from build123d import *

# Parameters (mm, degrees)
SKETCH_1_W          = 69
SKETCH_1_H          = 30
EXTRUDE_1_DEPTH     = 43
SKETCH_3_W          = 63
SKETCH_3_H          = 10
CUT_EXTRUDE_2_DEPTH = 41
SKETCH_4_W          = 69
SKETCH_4_H          = 17
CUT_EXTRUDE_3_DEPTH = 41
SKETCH_5_R          = 2.1
CUT_EXTRUDE_4_DEPTH = 56.643957444
SKETCH_9_W          = 55
SKETCH_9_H          = 30
CUT_EXTRUDE_5_DEPTH = 58.690987164
FILLET_1_R          = 3
FILLET_2_R          = 2
FILLET_3_R          = 1
SKETCH_10_W         = 8
SKETCH_10_H         = 30
CUT_EXTRUDE_6_DEPTH = 83.674058809
FILLET_4_R          = 1
FILLET_5_R          = 1


with BuildPart() as part:
    # 草图1 → 凸台-拉伸1 (new body)
    with BuildSketch(Plane(origin=(0, 0, 0), x_dir=(1, 0, 0), z_dir=(0, 1, 0))):
        Rectangle(SKETCH_1_W, SKETCH_1_H)
    extrude(amount=EXTRUDE_1_DEPTH)

    # 草图3 → 切除-拉伸2 (cut)
    with BuildSketch(Plane(origin=(0, 43, 0), x_dir=(1, 0, 0), z_dir=(0, 1, 0))):
        with Locations((-0.5, -10)):
            Rectangle(SKETCH_3_W, SKETCH_3_H)
    extrude(amount=-CUT_EXTRUDE_2_DEPTH, mode=Mode.SUBTRACT)

    # 草图4 → 切除-拉伸3 (cut)
    with BuildSketch(Plane(origin=(0, 0, 0), x_dir=(-1, 0, 0), z_dir=(0, -1, 0))):
        with Locations((0, 6.5)):
            Rectangle(SKETCH_4_W, SKETCH_4_H)
    extrude(amount=-CUT_EXTRUDE_3_DEPTH, mode=Mode.SUBTRACT)

    # 草图5 → 切除-拉伸4 (cut, through all)
    with BuildSketch(Plane(origin=(0, 41, 0), x_dir=(-1, 0, 0), z_dir=(0, -1, 0))):
        with Locations(Location((26.5, 7, 0), (0, 0, 90))):
            Circle(SKETCH_5_R)
    cut_extrude_4 = extrude(amount=-CUT_EXTRUDE_4_DEPTH, mode=Mode.SUBTRACT)

    # 镜向1: 切除-拉伸4 across plane
    add(cut_extrude_4.mirror(Plane.ZY), mode=Mode.SUBTRACT)

    # 草图9 → 切除-拉伸5 (cut, through all)
    with BuildSketch(Plane(origin=(0, 0, 2), x_dir=(-1, 0, 0), z_dir=(0, 0, -1))):
        with Locations((0, 20)):
            Rectangle(SKETCH_9_W, SKETCH_9_H)
    extrude(amount=-CUT_EXTRUDE_5_DEPTH, mode=Mode.SUBTRACT)

    # 圆角1
    fillet_1_edges = [part.edges().sort_by_distance(p)[0] for p in [
        (-27.5, 35, 3.5),
        (-27.5, 5, 3.5),
        (27.5, 5, 3.5),
        (27.5, 35, 3.5),
    ]]
    fillet(fillet_1_edges, radius=FILLET_1_R)

    # 圆角2
    fillet_2_edges = [part.edges().sort_by_distance(p)[0] for p in [
        (-34.5, 0, 8.5),
        (34.5, 0, 8.5),
        (-34.5, 42, -15),
        (34.5, 42, -15),
    ]]
    fillet(fillet_2_edges, radius=FILLET_2_R)

    # 圆角3
    fillet_3_edges = [part.edges().sort_by_distance(p)[0] for p in [
        (-32, 2, 10),
        (31, 2, 10),
    ]]
    fillet(fillet_3_edges, radius=FILLET_3_R)

    # 草图10 → 切除-拉伸6 (cut, through all)
    with BuildSketch(Plane.ZY.offset(34.5)):
        with Locations((6, 20.5)):
            Rectangle(SKETCH_10_W, SKETCH_10_H)
    extrude(amount=-CUT_EXTRUDE_6_DEPTH, mode=Mode.SUBTRACT)

    # 圆角4
    fillet_4_edges = [part.edges().sort_by_distance(p)[0] for p in [
        (31, 39.25, 5),
        (-32, 39.25, 5),
        (-33.25, 35.5, 10),
        (32.75, 35.5, 10),
        (32.75, 5.5, 10),
        (-33.25, 5.5, 10),
    ]]
    fillet(fillet_4_edges, radius=FILLET_4_R)

    # 圆角5
    fillet_5_edges = [part.edges().sort_by_distance(p)[0] for p in [
        (0, 0, 2),
        (33.914213562, 0.585786438, 2),
        (-33.914213562, 0.585786438, 2),
        (-34.5, 3.75, 2),
        (34.5, 3.75, 2),
        (-34.5, 38.25, 2),
        (34.5, 38.25, 2),
    ]]
    fillet(fillet_5_edges, radius=FILLET_5_R)


solid = part.part
Geometry: final body of the model. Coordinates: model frame, mm. A direction names the side the tool comes from. Round coordinates to 2 decimals unless told otherwise and drop trailing zeros. Loops run counter-clockwise (first coordinate to the right, second up) from the corner with the lowest first, then second, coordinate; pieces in that order, holes last.
Q1. Pin query (flat end, axial travel): P1, Ø14.5, axis at x = -11, z = -7.5, coming from the -Y side; P2, Ø5, axis at x = 12, y = 4, coming from the -Z side; P3, Ø1, axis at x = 33, y = 26, coming from the -Z side. Return the tip coordinate at first contact, or that it passes through.
Q2. Pull-direction query (X, two-part tool) for faces 4 (the cylindrical face through (33.93, 42.01, -14.4)), 5 (the flat face through (0, 43, -4)), 6 (the flat face through (31, 23, 12)); classes: released by +X, released by -X, zero draft, split by the parting line, or undercut.
Q3. Section A-A on x = -22. Return loops of the section in (y, z).
Q4. Material intervals for L1, parallel to X at y = 42, z = -7; L2, parallel to Z at x = 26.5, y = 42.35; L3, parallel to Y at x = -13, z = 0.5, sorted ascending.
Q5. Section B-B on z = -7. Return loops of the section in (x, y).
Q6. Section D-D on z = -1.5. Return loops of the section in (x, y).
Q7. Section C-C on y = 31.5. Return loops of the section in (x, z), plus the area to 3 significant figures.
Q8. Access query for faces 1 (the flat face through (0, 41, -6)), 2 (the flat face through (0, 5, 3)), 3 (the flat face through (-1, 2, 10)). Directions: +Z, -Z, +X, -X, +Y, -Y. A direction counts if a zero-diameter tool reaches every point of the face in a straight line with its end or side. Return the directions, or none.
Evaluation:
1. P1: stops at y = 41
1. P2: stops at z = 2
1. P3: stops at z = 10
2. face 4: released by +X
2. face 5: zero draft
2. face 6: undercut
3. outline: (0, 3) arc R1 ccw to (1, 2) - (5, 2) - (5, 5) - (2, 5) - (2, 15) - (0, 15) - close; (35.5, 2) - (41, 2) - (41, -15) - (43, -15) - (43, 5) - (35.5, 5) - close
4. L1: x = -34.5 to -28.6, -24.4 to 24.4, 28.6 to 34.5
4. L2: z = -15 to -9.1, -4.9 to 5
4. L3: y = 41 to 43
5. outline: (-34.5, 41) - (-28.6, 41) - (-28.6, 43) - (-34.5, 43) - close; (-24.4, 41) - (24.4, 41) - (24.4, 43) - (-24.4, 43) - close; (28.6, 41) - (34.5, 41) - (34.5, 43) - (28.6, 43) - close
6. outline: (-34.5, 41) - (34.5, 41) - (34.5, 43) - (-34.5, 43) - close
7. outline: (-34.5, 10) - (-32, 10) - (-32, 15) - (-34.5, 15) - close; (31, 10) - (34.5, 10) - (34.5, 15) - (31, 15) - close
7. area: 30.0 mm2
8. face 1: -Z, +X, -X, -Y
8. face 2: +Z, -Z
8. face 3: +Z, +Y
